from build123d import *

# Parameters (mm, degrees)
DODANIE_WYCI_GNI_CIE1_DEPTH = 1.5
ZAOKR_GLENIE1_R             = 4
SZKIC2_R                    = 1.5
WYTNIJ_WYCI_GNI_CIE1_DEPTH  = 197.62293997
SZYK_KO_OWY1_COUNT          = 4
WYTNIJ_WYCI_GNI_CIE2_REACH  = 198.623
SZYK_KO_OWY2_COUNT          = 4
WYTNIJ_WYCI_GNI_CIE3_REACH  = 198.623
SZKIC4_R                    = 2


with BuildPart() as part:
    # Szkic1 → Dodanie-wyci_gni_cie1 (new body)
    with BuildSketch(Plane(origin=(0, 0, 0), x_dir=(1, 0, 0), z_dir=(0, 1, 0))):
        with BuildLine():
            Line((-70, -140), (-140, -70))
            add(Edge.make_bspline(
                [(-140, 70), (-100, 0), (-140, -70)],
                knots=[0, 0, 0, 1, 1, 1], degree=2))
            Line((-140, 70), (-70, 140))
            add(Edge.make_bspline(
                [(70, 140), (0, 100), (-70, 140)],
                knots=[0, 0, 0, 1, 1, 1], degree=2))
            Line((70, 140), (140, 70))
            add(Edge.make_bspline(
                [(140, -70), (100, 0), (140, 70)],
                knots=[0, 0, 0, 1, 1, 1], degree=2))
            Line((140, -70), (70, -140))
            add(Edge.make_bspline(
                [(-70, -140), (0, -100), (70, -140)],
                knots=[0, 0, 0, 1, 1, 1], degree=2))
        make_face()
    extrude(amount=DODANIE_WYCI_GNI_CIE1_DEPTH)

    # Zaokr_glenie1
    zaokr_glenie1_edges = [part.edges().sort_by_distance(p)[0] for p in [
        (-140, 0.75, -70),
        (-70, 0.75, -140),
        (70, 0.75, -140),
        (140, 0.75, -70),
        (140, 0.75, 70),
        (70, 0.75, 140),
        (-140, 0.75, 70),
        (-70, 0.75, 140),
    ]]
    fillet(zaokr_glenie1_edges, radius=ZAOKR_GLENIE1_R)

    # Szkic2 → Wytnij-wyci_gni_cie1 (cut, through all)
    with BuildSketch(Plane(origin=(0, 1.5, 0), x_dir=(1, 0, 0), z_dir=(0, 1, 0))):
        with Locations(Location((-78.488852712, -119.501046021, 0), (0, 0, 270))):
            Circle(SZKIC2_R)
        with Locations(Location((-119.501046021, -78.488852712, 0), (0, 0, 90))):
            Circle(SZKIC2_R)
        with Locations(Location((-50.204581464, -91.216774773, 0), (0, 0, 90))):
            Circle(SZKIC2_R)
        with Locations(Location((-91.216774773, -50.204581464, 0), (0, 0, 270))):
            Circle(SZKIC2_R)
    wytnij_wyci_gni_cie1 = extrude(amount=-WYTNIJ_WYCI_GNI_CIE1_DEPTH, mode=Mode.SUBTRACT)

    # Szyk ko_owy1: Wytnij-wyci_gni_cie1 ×4 about axis
    szyk_ko_owy1_axis = Axis((0, 0, 0), (0, 1, 0))
    for i in range(1, SZYK_KO_OWY1_COUNT):
        add(wytnij_wyci_gni_cie1.rotate(szyk_ko_owy1_axis, i * 360 / SZYK_KO_OWY1_COUNT), mode=Mode.SUBTRACT)

    # Szkic3 → Wytnij-wyci_gni_cie2 (cut, up to next)
    with BuildSketch(Plane(origin=(0, 1.5, 0), x_dir=(1, 0, 0), z_dir=(0, 1, 0)), mode=Mode.PRIVATE) as wytnij_wyci_gni_cie2_sk1:
        with BuildLine():
            Line((-68.568652292, 56.387088824), (-47.355448856, 77.60029226))
            ThreePointArc((-47.355448856, 77.60029226), (-37.45595392, 77.60029226), (-37.45595392, 67.700797323))
            Line((-37.45595392, 67.700797323), (-58.669157355, 46.487593888))
            ThreePointArc((-58.669157355, 46.487593888), (-68.568652292, 46.487593888), (-68.568652292, 56.387088824))
        make_face()
    wytnij_wyci_gni_cie2_tool1 = extrude(wytnij_wyci_gni_cie2_sk1.sketch, amount=-WYTNIJ_WYCI_GNI_CIE2_REACH, mode=Mode.PRIVATE) & part.part
    wytnij_wyci_gni_cie2 = wytnij_wyci_gni_cie2_tool1.solids().sort_by_distance((-53.012303, 1.5, -62.043943))[0]
    add(wytnij_wyci_gni_cie2, mode=Mode.SUBTRACT)

    # Szyk ko_owy2: Wytnij-wyci_gni_cie2 ×4 about axis
    szyk_ko_owy2_axis = Axis((0, 0, 0), (0, 1, 0))
    for i in range(1, SZYK_KO_OWY2_COUNT):
        add(wytnij_wyci_gni_cie2.rotate(szyk_ko_owy2_axis, i * 360 / SZYK_KO_OWY2_COUNT), mode=Mode.SUBTRACT)

    # Szkic4 → Wytnij-wyci_gni_cie3 (cut, up to next)
    with BuildSketch(Plane(origin=(0, 1.5, 0), x_dir=(1, 0, 0), z_dir=(0, 1, 0)), mode=Mode.PRIVATE) as wytnij_wyci_gni_cie3_sk1:
        with Locations(Location((-68.34, 0, 0), (0, 0, 270))):
            Circle(SZKIC4_R)
    wytnij_wyci_gni_cie3_tool1 = extrude(wytnij_wyci_gni_cie3_sk1.sketch, amount=-WYTNIJ_WYCI_GNI_CIE3_REACH, mode=Mode.PRIVATE) & part.part
    # Szkic4 → Wytnij-wyci_gni_cie3 (cut, up to next)
    with BuildSketch(Plane(origin=(0, 1.5, 0), x_dir=(1, 0, 0), z_dir=(0, 1, 0)), mode=Mode.PRIVATE) as wytnij_wyci_gni_cie3_sk2:
        with Locations(Location((68.34, 0, 0), (0, 0, 270))):
            Circle(SZKIC4_R)
    wytnij_wyci_gni_cie3_tool2 = extrude(wytnij_wyci_gni_cie3_sk2.sketch, amount=-WYTNIJ_WYCI_GNI_CIE3_REACH, mode=Mode.PRIVATE) & part.part
    add(wytnij_wyci_gni_cie3_tool1.solids().sort_by_distance((-68.34, 1.5, 0))[0], mode=Mode.SUBTRACT)
    add(wytnij_wyci_gni_cie3_tool2.solids().sort_by_distance((68.34, 1.5, 0))[0], mode=Mode.SUBTRACT)


solid = part.part
Can you work these out from the model? Positions are in its coordinate system, mm. A direction names the side the tool comes from. Coordinates: 2 decimals unless noted, no trailing zeros. Loops run counter-clockwise (first coordinate to the right, second up) from the corner with the lowest first, then second, coordinate; pieces in that order, holes last. Notation, with made-up numbers: (7.25, 71) - (17.25, 71) arc R29 cw to (17.25, 98) - close; hole circle Ø6 at (-38, 79). An arc over 180 degrees is marked (long way). Answer as a JSON object with one key per item and string values. Group by question number.
Item 1: If we section it at C-C (y = 0.5): State how many separate pieces and enclosed holes the cut face has, plus the area to 3 significant figures.
Item 2: If we mould it in two halves opening along X, with no side actions, what happens to faces 3 (the face through (-105, 1, -105)), 4 (the face through (-37.57, 0.76, -77.71)), 5 (the face through (105, 1, -105)), 6 (the face through (-46.38, 0.76, 68.46))? For each: released by +X, released by -X, zero draft, split by the parting line, or undercut.
Item 3: If we section it at A-A (z = 106): List the corners of the cut face in (x, y) for me, plus the area to 3 significant figures.
Item 4: On a 3-axis mill with a long thin cutter (end or side, diameter ignored), from which of +Z, -Z, +X, -X, +Y, -Y can I reach the whole of each face in a straight line? I mean faces 1 (the face through (58.111, 0.76, 66.845)), 2 (the face through (105, 1, 105)). Say none if no direction works.
Item 5: If we section it at B-B (x = -114): List the corners of the cut face in (y, z) for me, plus the area to 3 significant figures.
Item 6: For pin 1 (1.8 mm diameter, centred on x = 50.2, z = -91.22, fed in from +Y); pin 2 (5 mm diameter, centred on x = -50.2, z = -91.22, fed in from -Y), each with a flat end and sliding along its axis, tell me the tip position at first contact or that it passes through.
Item 7: If I drill on L1, parallel to X at y = 0.5, z = 0; L2, parallel to Z at x = 54, y = 1.15; L3, parallel to Z at x = 52.5, y = 1.15, over which ranges is the centre line in solid material (lowest first)? Write a range as from..to.
Returned:
{
 "1": {"separate pieces": "1", "enclosed holes": "22", "area": "58,700 mm²"},
 "2": {"face 3": "released by -X", "face 4": "undercut", "face 5": "released by +X", "face 6": "undercut"},
 "3": {"outline": "(-104, 0) - (104, 0) - (104, 1.5) - (-104, 1.5) - close", "area": "312 mm²"},
 "4": {"face 1": "+Y, -Y", "face 2": "+Z, +X, +Y, -Y"},
 "5": {"outline": "(0, -96) - (1.5, -96) - (1.5, 96) - (0, 96) - close", "area": "288 mm²"},
 "6": {"pin 1": "passes through", "pin 2": "stops at y = 0"},
 "7": {"L1": "x = -120..-70.34, -66.34..66.34, 70.34..120", "L2": "z = -131.9..-70.13, -51.16..51.16, 70.96..131.9", "L3": "z = -131.25..-70.54, -52.66..52.66, 72.46..131.25"}
}
